```python
from build123d import *

# Parameters (mm, degrees)
F0_W     = 205.717654
F0_H     = 97.017468
F1_DEPTH = 2.54
F2_R     = 25.4
F3_R     = 4.435066
F4_DEPTH = 2.54


with BuildPart() as f1:
    # F0 (on Front) → F1 (new body)
    with BuildSketch(Plane.XZ):
        Rectangle(F0_W, F0_H)
    extrude(amount=F1_DEPTH)

    # F2
    f2_edges = [f1.edges().sort_by_distance(p)[0] for p in [
        (102.858827, -1.27, 48.508734),
        (102.858827, -1.27, -48.508734),
        (-102.858827, -1.27, -48.508734),
        (-102.858827, -1.27, 48.508734),
    ]]
    fillet(f2_edges, radius=F2_R)

    # F3 (on face) → F4 (cut)
    with BuildSketch(Plane.XZ.offset(2.54)):
        with Locations((-89.973114, -33.48276)):
            Circle(F3_R)
    extrude(amount=-F4_DEPTH, mode=Mode.SUBTRACT)


solid = f1.part
```
Could you check a few things on this model? Use its own coordinates, in mm. Give positions to 0.01 mm unless a question says otherwise; leave off trailing zeros. Order: outer loops, then holes, each group sorted by start corner. A loop starts at its lowest first (then second) coordinate and runs counter-clockwise, first axis right, second up.
Q1. If I drill on line 1 along X through (y, z) = (-0.55, -37); line 2 along X through (y, z) = (-0.25, -33.5); line 3 along X through (y, z) = (-2.3, 43.5), over which ranges is the centre line in solid material (lowest first)?
Q2. I'm going to push a flat-ended pin straight in: P1, Ø1.5, axis at y = -2, z = 31.5, coming from the -X side. Where does the tip first touch, or does it pass through?
Q3. Suppose I cut it at A-A, the plane y = -1.95. Write out the boundary of the cut face in (x, z), and give its area (3 significant figures).
Q4. Suppose I cut it at C-C, the plane x = 86.5. Write out the boundary of the cut face in (y, z), and give its area (3 significant figures).
Q5. We'd pull the mould along X, two halves only. Please class faces 1 (the cylindrical face through (95.616, -1.288, 40.871)), 2 (the flat face through (-1, -2.54, 1)), 3 (the cylindrical face through (-95.616, -1.288, -40.871)), 4 (the cylindrical face through (-90.935, -1.288, -37.812)): +X half, -X half, draft (parallel to the pull), parting line (faces both ways), or undercut.
Q6. Suppose I cut it at B-B, the plane z = 36. Write out the boundary of the cut face in (x, y).
Solution:
1. line 1: x = -98.72 to -92.67, -87.27 to 98.72
1. line 2: x = -100.64 to -94.41, -85.54 to 100.64
1. line 3: x = -92.6 to 92.6
2. P1: stops at x = -101.68
3. outline: (-102.86, -23.11) arc R25.4 ccw to (-77.46, -48.51) - (77.46, -48.51) arc R25.4 ccw to (102.86, -23.11) - (102.86, 23.11) arc R25.4 ccw to (77.46, 48.51) - (-77.46, 48.51) arc R25.4 ccw to (-102.86, 23.11) - close; hole circle Ø8.87 at (-89.97, -33.48)
3. area: 19,300 mm2
4. outline: (-2.54, -46.85) - (0, -46.85) - (0, 46.85) - (-2.54, 46.85) - close
4. area: 238 mm2
5. face 1: +X half
5. face 2: draft
5. face 3: -X half
5. face 4: undercut
6. outline: (-99.34, -2.54) - (99.34, -2.54) - (99.34, 0) - (-99.34, 0) - close
